from build123d import *

# Parameters (mm, degrees)
F0_W     = 24
F0_H     = 24
F1_DEPTH = 18.9
F1_TAPER = 10
F2_R     = 4.7910842269
F3_DEPTH = 45.7


with BuildPart() as f1:
    # F0 (on Top) → F1 (new body)
    with BuildSketch(Plane.XY):
        Rectangle(F0_W, F0_H)
    extrude(amount=F1_DEPTH, taper=F1_TAPER)

    # F2 (on face) → F3 (join)
    with BuildSketch(Plane.XY.offset(18.9)):
        Circle(F2_R)
    extrude(amount=F3_DEPTH)

    # F4 (on Front) → F5 (revolve)
    with BuildSketch(Plane.XZ):
        Polygon((0, 92.3125015855), (0, 64.6), (17.6069048751, 64.6), (33.799842, 92.3125015855), align=None)
    revolve(axis=Axis((0, 0, 78.4562507927), (0, 0, -1)))


solid = f1.part
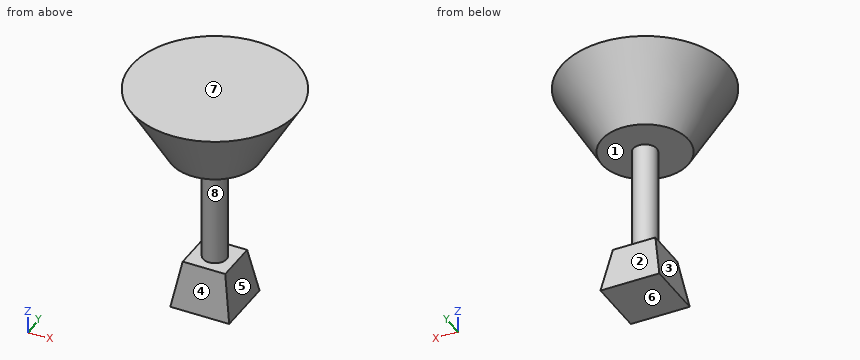
Input: part model. Units: mm. Frame: model coordinates. Face numbers are marked on the shaded views. A direction names the side the tool comes from. Coordinates: 2 decimals unless noted, no trailing zeros. Order: outer loops, then holes, each group sorted by start corner. A loop starts at its lowest first (then second) coordinate and runs counter-clockwise, first axis right, second up.
1. Cut plane C-C, the plane z = 37.5. Return loops of the section in (x, y).
Checked values:
outline: circle Ø9.58 at (0, 0)
2. Cut plane D-D, the plane z = 17. Return loops of the section in (x, y), plus the area to 3 significant figures.
Checked values:
outline: (-9, -9) - (9, -9) - (9, 9) - (-9, 9) - close
area: 324 mm2
3. Cut plane A-A, the plane x = 0. Return loops of the section in (y, z), plus the area to 3 significant figures.
Checked values:
outline: (-33.8, 92.31) - (-17.61, 64.6) - (-4.79, 64.6) - (-4.79, 18.9) - (-8.67, 18.9) - (-12, 0) - (12, 0) - (8.67, 18.9) - (4.79, 18.9) - (4.79, 64.6) - (17.61, 64.6) - (33.8, 92.31) - close
area: 2,250 mm2
4. Access query for the marked faces 1, 2, 3, 4 and 5. Directions: +Z, -Z, +X, -X, +Y, -Y. A direction counts if a zero-diameter tool reaches every point of the face in a straight line with its end or side. Return the directions, or none.
Checked values:
face 1: none
face 2: +X, -X, +Y
face 3: -X, +Y, -Y
face 4: +X, -X, -Y
face 5: +X, +Y, -Y
5. Draft query along Z for the marked faces 6, 7 and 8. Return one class per face: +Z half, -Z half, draft (parallel to the pull), parting line (faces both ways), or undercut.
Checked values:
face 6: -Z half
face 7: +Z half
face 8: undercut
6. Ray query, line 1 along Y through (x, z) = (-23.5, 79); line 2 along Y through (x, z) = (-3.5, 37.5); line 3 along Z through (x, y) = (1, -28). Return the intervals inside material, ascending.
Checked values:
line 1: y = -11.17 to 11.17
line 2: y = -3.27 to 3.27
line 3: z = 82.42 to 92.31
7. Contact query for flat-ended pins moving along their axis: P1, Ø12, axis at x = -20, y = -1.5, coming from the -Z side; P2, Ø8, axis at x = -15, z = 69, coming from the +Y side. Output: stop coordinate, or through.
Checked values:
P1: stops at z = 64.6
P2: stops at y = 18.12
